The model under review builds one solid part; all positions refer to its coordinate system, in mm. A direction names the side the tool comes from. Coordinates: 2 decimals unless noted, no trailing zeros. Write each loop counter-clockwise with the first axis right and the second up, starting at its lowest first coordinate (ties: lowest second). Pieces come first, ordered by that corner, then holes. Notation, with made-up numbers: (-3.75, 11) - (28.25, 11) arc R19 ccw to (28.25, 31) - close; hole circle Ø5 at (-7.5, 6). An arc over 180 degrees is marked (long way). Return JSON: item names as keys, results as strings. Group by question number.
(1) For pin 1 Ø1 at (x, y) = (7.5, 2) entering from +Z; pin 2 Ø12 at (x, z) = (-7, 3.5) entering from -Y; pin 3 Ø3 at (x, y) = (19.5, 3.5) entering from -Z, all flat-tipped, find the tip position at first contact; note any pin that passes through.
(2) We need section B-B on z = 0. State the section outline as (x, y) points, then the cut area to 3 significant figures.
(3) We need section A-A on x = 0. State the section outline as (y, z) points.
(4) Draft analysis for pull direction X (two halves, no side actions). For faces 1 (the face through (7.509, 2.712, 23.846)), 2 (the face through (7.21, 1.73, -22.89)), 3 (the face through (0, 5.5, 0)), state which applies: released by +X, released by -X, zero draft, split by the parting line, or undercut.
(5) Tool access review of faces 4 (the face through (-18, 3.5, 11)), 5 (the face through (9.4, 0, -22.3)): name each direction out of +Z, -Z, +X, -X, +Y, -Y from which nothing blocks a thin tool from reaching the whole face with its end or side.
(6) To check wall thickness, follow L1, parallel to X at y = 3.85, z = 0; L2, parallel to X at y = 2.45, z = 0; L3, parallel to Y at x = 3, z = -17. State the ranges of each line that lie inside material, in increasing order. Write a range as from..to.
(7) We need section C-C on y = 2. State the section outline as (x, z) points, then the cut area to 3 significant figures.
```python
from build123d import *

# Parameters (mm, degrees)
SKETCH1_R           = 25
BOSS_EXTRUDE1_DEPTH = 5.5
SKETCH2_R           = 24
CUT_EXTRUDE1_DEPTH  = 3.5
SKETCH3_R           = 20.4
SKETCH3_R_2         = 19.9
CUT_EXTRUDE2_DEPTH  = 1


with BuildPart() as part:
    # Sketch1 → Boss-Extrude1 (new body)
    with BuildSketch(Plane(origin=(0, 0, 0), x_dir=(1, 0, 0), z_dir=(0, 1, 0))):
        with Locations(Location((0, 0, 0), (0, 0, 270))):
            Circle(SKETCH1_R)
    extrude(amount=BOSS_EXTRUDE1_DEPTH)

    # Sketch2 → Cut-Extrude1 (cut)
    with BuildSketch(Plane.XZ):
        with Locations(Location((0, 0, 0), (0, 0, 270))):
            Circle(SKETCH2_R)
    extrude(amount=-CUT_EXTRUDE1_DEPTH, mode=Mode.SUBTRACT)

    # Sketch3 → Cut-Extrude2 (cut)
    with BuildSketch(Plane(origin=(0, 3.5, 0), x_dir=(-1, 0, 0), z_dir=(0, -1, 0))):
        with Locations(Location((0, 0, 0), (0, 0, 90))):
            Circle(SKETCH3_R)
        with Locations(Location((0, 0, 0), (0, 0, 90))):
            Circle(SKETCH3_R_2, mode=Mode.SUBTRACT)
    extrude(amount=-CUT_EXTRUDE2_DEPTH, mode=Mode.SUBTRACT)


solid = part.part
```
Ans:
{
 "1": {"pin 1": "z = 24", "pin 2": "y = 3.5", "pin 3": "z = -17.35"},
 "2": {"outline": "(-25, 0) - (-24, 0) - (-24, 3.5) - (-20.4, 3.5) - (-20.4, 4.5) - (-19.9, 4.5) - (-19.9, 3.5) - (19.9, 3.5) - (19.9, 4.5) - (20.4, 4.5) - (20.4, 3.5) - (24, 3.5) - (24, 0) - (25, 0) - (25, 5.5) - (-25, 5.5) - close", "area": "106 mm²"},
 "3": {"outline": "(0, -25) - (5.5, -25) - (5.5, 25) - (0, 25) - (0, 24) - (3.5, 24) - (3.5, 20.4) - (4.5, 20.4) - (4.5, 19.9) - (3.5, 19.9) - (3.5, -19.9) - (4.5, -19.9) - (4.5, -20.4) - (3.5, -20.4) - (3.5, -24) - (0, -24) - close"},
 "4": {"face 1": "split by the parting line", "face 2": "undercut", "face 3": "zero draft"},
 "5": {"face 4": "-Y", "face 5": "+Z, -Z, +X, -X, -Y"},
 "6": {"L1": "-25..-20.4, -19.9..19.9, 20.4..25", "L2": "-25..-24, 24..25", "L3": "3.5..5.5"},
 "7": {"outline": "circle Ø50 at (0, 0); hole circle Ø48 at (0, 0)", "area": "154 mm²"}
}
